```python
from build123d import *

# Parameters (mm, degrees)
F0_W     = 203.2
F0_H     = 101.6
F1_DEPTH = 101.6


with BuildPart() as f1:
    # F0 (on Front) → F1 (new body)
    with BuildSketch(Plane.XZ):
        Rectangle(F0_W, F0_H)
        Polygon((82.55, 44.45), (95.25, 44.45), (95.25, 19.05), (95.25, -44.45), (0, -44.45), (-95.25, -44.45), (-95.25, 44.45), (0, 44.45), align=None, mode=Mode.SUBTRACT)
    extrude(amount=F1_DEPTH)


solid = f1.part
```
Verification items for the finished model (mm, model axes). A direction names the side the tool comes from. Give positions to 0.01 mm unless a question says otherwise; leave off trailing zeros. Order: outer loops, then holes, each group sorted by start corner. A loop starts at its lowest first (then second) coordinate and runs counter-clockwise, first axis right, second up. Notation, with made-up numbers: (84, 26) -> (95, 26) arc R18 cw to (95, 34) -> close; hole circle Ø1 at (-34.75, 49). An arc over 180 degrees is marked (long way). One line per item, written item: value.
(1) Tool access check on faces 4 (the face through (95.25, -50, 1)), 5 (the face through (-8, -101.6, -45)). Record the directions out of +Z, -Z, +X, -X, +Y, -Y that give a thin tool (end or side, any length) a straight path to the whole face; none if there is none.
Final values:
face 4: +Y, -Y
face 5: +Z, -Z, +X, -X, -Y
(2) Sectioned sample at C-C on z = -32. Record the cut outline in (x, y), then the cut area to 3 significant figures.
Final values:
outline: (-101.6, -101.6) -> (-95.25, -101.6) -> (-95.25, 0) -> (-101.6, 0) -> close; (95.25, -101.6) -> (101.6, -101.6) -> (101.6, 0) -> (95.25, 0) -> close
area: 1,290 mm^2
(3) Sectioned sample at B-B on x = -59.5. Record the cut outline in (y, z), then the cut area to 3 significant figures.
Final values:
outline: (-101.6, -50.8) -> (0, -50.8) -> (0, -44.45) -> (-101.6, -44.45) -> close; (-101.6, 44.45) -> (0, 44.45) -> (0, 50.8) -> (-101.6, 50.8) -> close
area: 1,290 mm^2
(4) Scan lines: line 1 along Z through (x, y) = (30, -36); line 2 along X through (y, z) = (-11, -1.5). Record each from-to range of solid material in increasing order. Write a range as [from, to].
Final values:
line 1: [-50.8, -44.45], [44.45, 50.8]
line 2: [-101.6, -95.25], [95.25, 101.6]
(5) Draft check along Z on faces 1 (the face through (-95.25, -50, -1)), 2 (the face through (-1, -50, 50.8)), 3 (the face through (-1, -50, -50.8)). Enter one of: pulls with the +Z half, pulls with the -Z half, needs draft (parallel to the pull), parting line crosses it, or undercut.
Final values:
face 1: undercut
face 2: pulls with the +Z half
face 3: pulls with the -Z half
(6) Sectioned sample at A-A on y = -90.5. Record the cut outline in (x, z), then the cut area to 3 significant figures.
Final values:
outline: (-101.6, -50.8) -> (101.6, -50.8) -> (101.6, 50.8) -> (-101.6, 50.8) -> close; hole (-95.25, -44.45) -> (95.25, -44.45) -> (95.25, 44.45) -> (-95.25, 44.45) -> close
area: 3,710 mm^2
